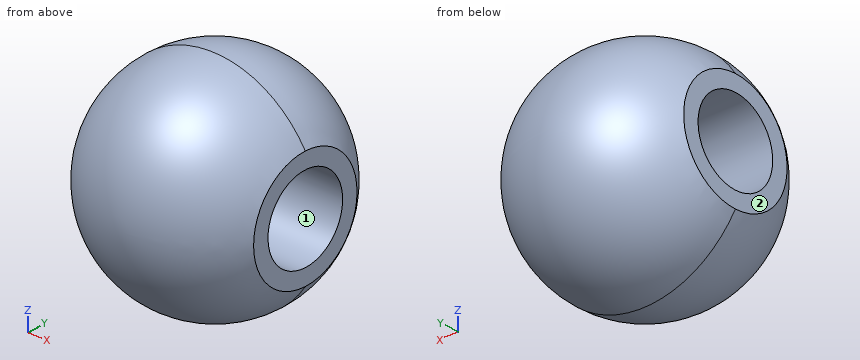
```python
from build123d import *

# Parameters (mm, degrees)
CUT_EXTRUDE3_DEPTH      = 5.5033321
CUT_EXTRUDE3_DEPTH_BACK = 5.5033321
SKETCH5_W               = 0.4
SKETCH5_H               = 8.681299001
SKETCH6_R               = 1
CUT_EXTRUDE5_DEPTH      = 6.734108475


with BuildPart() as part:
    # Sketch1 one side → Revolve5 (revolve)
    with BuildSketch(Plane.XY):
        with BuildLine():
            ThreePointArc((0, -2.6), (1.838477631, -1.838477631), (2.6, 0))
            ThreePointArc((2.6, 0), (1.838477631, 1.838477631), (0, 2.6))
            Line((0, 2.6), (0, -2.6))
        make_face()
    revolve(axis=Axis((0, 2.6, 0), (0, -1, 0)))

    # Sketch5 → Cut-Extrude3 (cut, two sides: drawn at the far end of the back side and taken through both)
    with BuildSketch(Plane.XY.offset(-CUT_EXTRUDE3_DEPTH_BACK)):
        with Locations((-2.4, -0.428203102)):
            Rectangle(SKETCH5_W, SKETCH5_H)
        with Locations((2.4, -0.428203102)):
            Rectangle(SKETCH5_W, SKETCH5_H)
    extrude(amount=CUT_EXTRUDE3_DEPTH + CUT_EXTRUDE3_DEPTH_BACK, mode=Mode.SUBTRACT)

    # Sketch6 → Cut-Extrude5 (cut, through all)
    with BuildSketch(Plane(origin=(2.2, 0, 0), x_dir=(0, 0, -1), z_dir=(1, 0, 0))):
        Circle(SKETCH6_R)
    extrude(amount=-CUT_EXTRUDE5_DEPTH, mode=Mode.SUBTRACT)


solid = part.part
```
The model under review builds one solid part; all positions refer to its coordinate system, in mm. Face numbers are marked on the shaded views. Give positions to 0.01 mm unless a question says otherwise; leave off trailing zeros. Write each loop counter-clockwise with the first axis right and the second up, starting at its lowest first coordinate (ties: lowest second). Pieces come first, ordered by that corner, then holes.
(1) For P1, Ø1, axis at x = 0.5, z = -1, coming from the +Y side, flat-tipped, find the tip position at first contact; note if it passes through.
(2) To check wall thickness, follow L1, parallel to Y at x = 1.25, z = 0; L2, parallel to Y at x = -0.05, z = -0.55; L3, parallel to Z at x = 1.85, y = 0.2. State the ranges of each line that lie inside material, in increasing order.
(3) Consider section C-C, the plane x = -1.3. Give the boundary of the cut face in (y, z), and give its area (3 significant figures).
(4) The part is to be moulded in two halves that separate along Y. For the marked faces 1 and 2, say which applies: released by +Y, released by -Y, zero draft, split by the parting line, or undercut.
(5) Consider section D-D, the plane z = 1.25. Give the boundary of the cut face in (x, y).
(6) Consider section A-A, the plane z = 0. Give the boundary of the cut face in (x, y), and give its area (3 significant figures).
(7) Consider section B-B, the plane y = -0.75. Give the boundary of the cut face in (x, z).
Returned:
1. P1: stops at y = 2.53
2. L1: y = -2.28 to -1, 1 to 2.28
2. L2: y = -2.54 to -0.84, 0.84 to 2.54
2. L3: z = -1.82 to -0.98, 0.98 to 1.82
3. outline: circle Ø4.5 at (0, 0); hole circle Ø2 at (0, 0)
3. area: 12.8 mm2
4. face 1: undercut
4. face 2: zero draft
5. outline: (-2.2, -0.6) arc R2.28 ccw to (2.2, -0.6) - (2.2, 0.6) arc R2.28 ccw to (-2.2, 0.6) - close
6. outline: (-2.2, -1.39) arc R2.6 ccw to (2.2, -1.39) - (2.2, -1) - (-2.2, -1) - close; (-2.2, 1) - (2.2, 1) - (2.2, 1.39) arc R2.6 ccw to (-2.2, 1.39) - close
6. area: 10.9 mm2
7. outline: (-2.2, -1.17) arc R2.49 ccw to (2.2, -1.17) - (2.2, -0.66) - (-2.2, -0.66) - close; (-2.2, 0.66) - (2.2, 0.66) - (2.2, 1.17) arc R2.49 ccw to (-2.2, 1.17) - close
